Autodesk Fusion 360 part; units mm, degrees
sketch "Sketch1" plane through (0, 0, 0) normal (0, 0, 1) x (1, 0, 0)
  line L0 (0, 0) -> (6.9, 0)
  line L1 (6.9, 0) -> (6.9, -2.1)
  line L2 (6.9, -2.1) -> (4.6, -2.1)
  line L3 (4.6, -2.1) -> (4.6, -3.1)
  line L4 (4.6, -3.1) -> (6.9335, -5.4335)
  line L5 (4.6, -3.1) -> (7.9, -3.1) construction
  line L6 (4.6, -2.1) -> (10.8, -2.1)
  line L7 (6.9, -2.1) -> (13.1, -2.1)
  line L8 (13.1, -2.1) -> (15.4, -2.1)
  line L9 (15.4, -2.1) -> (15.4, -3.1)
  line L10 (15.4, -3.1) -> (13.0665, -5.4335)
  line L11 (13.0665, -5.4335) -> (6.9335, -5.4335)
  line L12 (15.4, -2.1) -> (13.1, -2.1)
  line L13 (13.1, -2.1) -> (13.1, 0)
  line L14 (13.1, 0) -> (16.1, 0)
  line L15 (16.1, 0) -> (16.1, 2)
  line L16 (16.1, 2) -> (0, 2)
  line L17 (0, 2) -> (0, 0)
  dimension "d1" = 6.9
  dimension "d2" = 2.1
  dimension "d3" = 2.3
  dimension "d4" = 1
  dimension "d5" = 45
  dimension "d6" = 3.3
  dimension "d7" = 6.2
  dimension "d11" = 6.2
  dimension "d12" = 135
  dimension "d13" = 3.3
  dimension "d14" = 3
extrude "Extrude1" add sketch "Sketch1" along normal blind 68
sketch "Sketch11" plane through (0, -5.4335, 0) normal (0, -1, 0) x (1, 0, 0)
  line L0 (6.9335, 0) -> (13.0665, 0)
  line L1 (13.0665, 0) -> (13.0665, 68)
  line L2 (13.0665, 68) -> (6.9335, 68)
  line L3 (6.9335, 68) -> (6.9335, 0)
  circle A0 centre (9.9608, 60) radius 1.475
  dimension "d119" = 2.95
  dimension "d126" = 8
extrude "Extrude33" cut sketch "Sketch11" against normal blind 10 contours A0
pattern_linear "R-Pattern1" count 3 spacing 26 along (0, 0, -1) of "Extrude33"
sketch "Sketch12" plane through (0, -5.4335, 0) normal (0, -1, 0) x (1, 0, 0)
  circle A0 centre (9.9713, 60.0289) radius 3
  dimension "d127" = 6
extrude "Extrude34" cut sketch "Sketch12" against normal blind 2.2
pattern_linear "R-Pattern2" count 3 spacing 26 along (0, 0, -1) of "Extrude34"
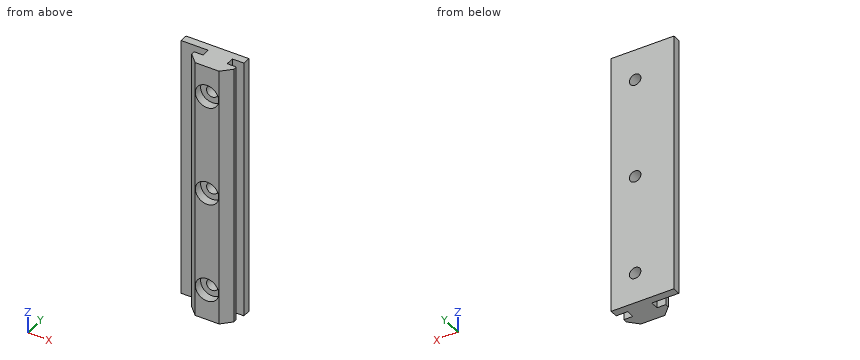
Can you work these out from the model? Positions are in its coordinate system, mm. Coordinates: 2 decimals unless noted, no trailing zeros. Write each loop counter-clockwise with the first axis right and the second up, starting at its lowest first coordinate (ties: lowest second). Pieces come first, ordered by that corner, then holes. Notation, with made-up numbers: (47.5, -23) -> (92.5, -23) arc R8 ccw to (92.5, -15) -> close; hole circle Ø2 at (53.5, -35). An arc over 180 degrees is marked (long way). Write item = value, one per line.
(1) For pin 1 (3.5 mm diameter, centred on x = 9.96, z = 8, fed in from -Y); pin 2 (1 mm diameter, centred on x = 2, z = 18.5, fed in from -Y); pin 3 (4 mm diameter, centred on x = 3.5, z = 52.5, fed in from -Y), each with a flat end and sliding along its axis, tell me the tip position at first contact or that it passes through.
Verdict:
pin_1 = -3.23
pin_2 = 0
pin_3 = -4
(2) Imagine slicing it at B-B (z = 14). Please give me the cut outline in (x, y).
Verdict:
outline = (0, 0) -> (6.9, 0) -> (6.9, -2.1) -> (4.6, -2.1) -> (4.6, -3.1) -> (6.93, -5.43) -> (13.07, -5.43) -> (15.4, -3.1) -> (15.4, -2.1) -> (13.1, -2.1) -> (13.1, 0) -> (16.1, 0) -> (16.1, 2) -> (0, 2) -> close
(3) If I drill on probe 1 along Z at (x, y) = (7.25, -4.25); probe 2 along Z at (x, y) = (8.75, -0.5); probe 3 along X at (y, z) = (-0.25, 51), over which ranges is the centre line in solid material (lowest first)?
Verdict:
probe_1 = 0 to 6.77, 9.29 to 32.77, 35.29 to 58.77, 61.29 to 68
probe_2 = 0 to 7.16, 8.84 to 33.16, 34.84 to 59.16, 60.84 to 68
probe_3 = 6.9 to 13.1
(4) Imagine slicing it at A-A (y = -1.25). Please give me the cut outline in (x, z) (3 decimals).
Verdict:
outline = (6.9, 0) -> (13.1, 0) -> (13.1, 68) -> (6.9, 68) -> close; hole circle Ø2.95 at (9.961, 8); hole circle Ø2.95 at (9.961, 34); hole circle Ø2.95 at (9.961, 60)
